Could you check a few things on this model? Use its own coordinates, in mm. Face numbers are marked on the shaded views. A direction names the side the tool comes from. Round coordinates to 2 decimals unless told otherwise and drop trailing zeros. Write each loop counter-clockwise with the first axis right and the second up, starting at its lowest first coordinate (ties: lowest second). Pieces come first, ordered by that corner, then holes. Notation, with made-up numbers: (-7.75, 26) -> (39.25, 26) arc R18 ccw to (39.25, 34) -> close; hole circle Ø2 at (34, -22.5). An arc over 180 degrees is marked (long way). Answer in a Markdown table with one row per item.
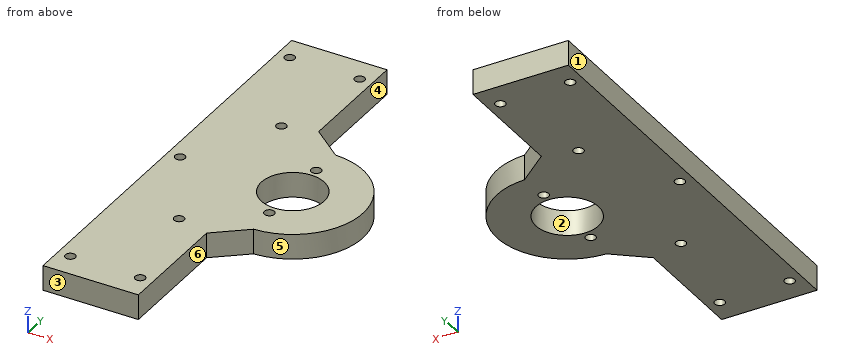
from build123d import *

# Parameters (mm, degrees)
SKETCH1_R           = 2
SKETCH1_R_2         = 12.5
BOSS_EXTRUDE1_DEPTH = 10


with BuildPart() as part:
    # Sketch1 → Boss-Extrude1 (new body)
    with BuildSketch(Plane.XY):
        with BuildLine():
            Line((-1.000028724, -38.297888442), (11.718065373, -27.990486171))
            ThreePointArc((11.718065373, -27.990486171), (39.000028724, 0.00030559), (11.718065373, 27.99109735))
            Line((11.718065373, 27.99109735), (-1.000028724, 38.298499621))
            Line((-1.000028724, 38.298499621), (-1.000028724, 85))
            Line((-1.000028724, 85), (-39.000028724, 85))
            Line((-39.000028724, 85), (-39.000028724, -85))
            Line((-39.000028724, -85), (-1.000028724, -85))
            Line((-1.000028724, -85), (-1.000028724, -38.297888442))
        make_face()
        with Locations((-13.916259829, -35)):
            Circle(SKETCH1_R, mode=Mode.SUBTRACT)
        with Locations((-13.916259829, 35)):
            Circle(SKETCH1_R, mode=Mode.SUBTRACT)
        with Locations((11.000028724, 0.00030559)):
            Circle(SKETCH1_R_2, mode=Mode.SUBTRACT)
        with Locations((-6.083797619, 75)):
            Circle(SKETCH1_R, mode=Mode.SUBTRACT)
        with Locations((-6.083797619, -75)):
            Circle(SKETCH1_R, mode=Mode.SUBTRACT)
        with Locations((-33.916259829, 75)):
            Circle(SKETCH1_R, mode=Mode.SUBTRACT)
        with Locations((-33.916259829, 0)):
            Circle(SKETCH1_R, mode=Mode.SUBTRACT)
        with Locations((11.000028724, -15.99969441)):
            Circle(SKETCH1_R, mode=Mode.SUBTRACT)
        with Locations((11.000028724, 16.00030559)):
            Circle(SKETCH1_R, mode=Mode.SUBTRACT)
        with Locations((-33.916259829, -75)):
            Circle(SKETCH1_R, mode=Mode.SUBTRACT)
    extrude(amount=BOSS_EXTRUDE1_DEPTH)


solid = part.part
1) Imagine slicing it at C-C, the plane z = 3. Count the separate pieces of the cut face and the enclosed holes in it, plus the area to 3 significant figures.
Findings:
| item | result |
|---|---|
| separate pieces | 1 |
| enclosed holes | 10 |
| area | 7,890 mm^2 |
2) For the marked faces 5 and 6, which set-ups out of +Z, -Z, +X, -X, +Y, -Y let a thin tool reach every point of the face, with its end or its side?
Findings:
| item | result |
|---|---|
| face 5 | +Z, -Z, +X |
| face 6 | +Z, -Z, +X, -Y |
3) Imagine slicing it at A-A, the plane y = 75. Please give me the cut outline in (x, z).
Findings:
| item | result |
|---|---|
| outline | (-39, 0) -> (-35.92, 0) -> (-35.92, 10) -> (-39, 10) -> close; (-31.92, 0) -> (-8.08, 0) -> (-8.08, 10) -> (-31.92, 10) -> close; (-4.08, 0) -> (-1, 0) -> (-1, 10) -> (-4.08, 10) -> close |
4) Please list where these lines run through material, in increasing order: line 1 (Y direction, x = 10, z = 5.5); line 2 (X direction, y = 46.5, z = 6); line 3 (Y direction, x = -13.5, z = 8.75).
Findings:
| item | result |
|---|---|
| line 1 | y = -29.38 to -17.73, -14.27 to -12.46, 12.46 to 14.27, 17.73 to 29.38 |
| line 2 | x = -39 to -1 |
| line 3 | y = -85 to -36.96, -33.04 to 33.04, 36.96 to 85 |
5) For pin 1 (5 mm diameter, centred on y = -69, z = 7, fed in from +X); pin 2 (5 mm diameter, centred on x = 20.5, z = 5.5, fed in from -Y); pin 3 (1 mm diameter, centred on x = 15, z = 3.5, fed in from -Y), each with a flat end and sliding along its axis, tell me the tip position at first contact or that it passes through.
Findings:
| item | result |
|---|---|
| pin 1 | stops at x = -1 |
| pin 2 | stops at y = -27.11 |
| pin 3 | stops at y = -27.78 |
6) Imagine slicing it at B-B, the plane x = 18. Please give me the cut outline in (y, z).
Findings:
| item | result |
|---|---|
| outline | (-27.11, 0) -> (-10.36, 0) -> (-10.36, 10) -> (-27.11, 10) -> close; (10.36, 0) -> (27.11, 0) -> (27.11, 10) -> (10.36, 10) -> close |
7) Thinking about a two-plate mould opening in X: for the marked faces 1, 2, 3 and 4, which applies, +X half, -X half, draft (parallel to the pull), parting line (faces both ways), or undercut?
Findings:
| item | result |
|---|---|
| face 1 | -X half |
| face 2 | undercut |
| face 3 | draft |
| face 4 | +X half |
8) Imagine slicing it at D-D, the plane y = 35. Please give me the cut outline in (x, z), plus the area to 3 significant figures.
Findings:
| item | result |
|---|---|
| outline | (-39, 0) -> (-15.92, 0) -> (-15.92, 10) -> (-39, 10) -> close; (-11.92, 0) -> (3.07, 0) -> (3.07, 10) -> (-11.92, 10) -> close |
| area | 381 mm^2 |
